from build123d import *

# Parameters (mm, degrees)
F0_R     = 8
F1_DEPTH = 37
F2_R     = 1.5
F3_DEPTH = 8
F6_DEPTH = 24.046


with BuildPart() as f1:
    # F0 (on Top) → F1 (new body)
    with BuildSketch(Plane.XY):
        Circle(F0_R)
    extrude(amount=F1_DEPTH)

    # F2 (on face) → F3 (join)
    with BuildSketch(Plane(origin=(0, 0, 0), x_dir=(1, 0, 0), z_dir=(0, 0, -1))):
        Circle(F2_R)
    extrude(amount=F3_DEPTH)

    # F5 (on face) → F6 (cut, through all)
    with BuildSketch(Plane.XY.offset(37)):
        with BuildLine():
            Line((-6.4125, -4.783288), (-6.4125, 4.783288))
            ThreePointArc((-6.4125, 4.783288), (-8, 0), (-6.4125, -4.783288))
        make_face()
        with BuildLine():
            ThreePointArc((6.4125, -4.783288), (8, 0), (6.4125, 4.783288))
            Line((6.4125, 4.783288), (6.4125, -4.783288))
        make_face()
    extrude(amount=-F6_DEPTH, mode=Mode.SUBTRACT)


solid = f1.part
Input: part model. Units: mm. Frame: model coordinates. A direction names the side the tool comes from. Coordinates: 2 decimals unless noted, no trailing zeros. Loops run counter-clockwise (first coordinate to the right, second up) from the corner with the lowest first, then second, coordinate; pieces in that order, holes last. Notation, with made-up numbers: (88.25, 85) -> (94.25, 85) arc R24 ccw to (94.25, 118) -> close; hole circle Ø4 at (-40, 84). An arc over 180 degrees is marked (long way). Write item = value, one per line. Start each with the question number.
Item 1: First-contact query: P1, Ø3, axis at y = 2.5, z = 6, coming from the -X side; P2, Ø5, axis at y = 1.5, z = 29.5, coming from the +X side; P3, Ø6, axis at x = -4, z = 7.5, coming from the +Y side. Flat tips, straight axial feed; report the tip coordinate or a pass-through.
Item 2: Material intervals for line 1 (Z direction, x = 1.25, y = 1.25); line 2 (X direction, y = -1, z = 29.5); line 3 (X direction, y = -3.75, z = 2), sorted ascending.
Item 3: Cut plane C-C, the plane z = 17.5. Return loops of the section in (x, y), plus the area to 3 significant figures.
Item 4: Cut plane A-A, the plane x = 0. Return loops of the section in (y, z).
Item 5: Cut plane D-D, the plane y = 3.75. Return loops of the section in (x, z).
Item 6: Reachability of faces 1 (the face through (-5.9, 5.4, 18.2)), 2 (the face through (-7, 0, 12.954)), 3 (the face through (-1.5, -0.07, -3.94)), 4 (the face through (7, 0, 12.954)), 5 (the face through (0, 0, -8)) from +Z, -Z, +X, -X, +Y, -Y: full face, straight path, thin tool, end or side. Return the list, or none.
Item 7: Cut plane B-B, the plane y = 0. Return loops of the section in (x, z), plus the area to 3 significant figures.
Ans:
q1.P1 = -7.94
q1.P2 = 6.41
q1.P3 = 7.94
q2.line_1 = 0 to 37
q2.line_2 = -6.41 to 6.41
q2.line_3 = -7.07 to 7.07
q3.outline = (-6.41, -4.78) arc R8 ccw to (6.41, -4.78) -> (6.41, 4.78) arc R8 ccw to (-6.41, 4.78) -> close
q3.area = 180 mm²
q4.outline = (-8, 0) -> (-1.5, 0) -> (-1.5, -8) -> (1.5, -8) -> (1.5, 0) -> (8, 0) -> (8, 37) -> (-8, 37) -> close
q5.outline = (-7.07, 0) -> (7.07, 0) -> (7.07, 12.95) -> (6.41, 12.95) -> (6.41, 37) -> (-6.41, 37) -> (-6.41, 12.95) -> (-7.07, 12.95) -> close
q6.face_1 = +Z, -Z
q6.face_2 = +Z, -X, +Y, -Y
q6.face_3 = -Z
q6.face_4 = +Z, +X, +Y, -Y
q6.face_5 = -Z, +X, -X, +Y, -Y
q7.outline = (-8, 0) -> (-1.5, 0) -> (-1.5, -8) -> (1.5, -8) -> (1.5, 0) -> (8, 0) -> (8, 12.95) -> (6.41, 12.95) -> (6.41, 37) -> (-6.41, 37) -> (-6.41, 12.95) -> (-8, 12.95) -> close
q7.area = 540 mm²
